Could you check a few things on this model? Use its own coordinates, in mm. Face numbers are marked on the shaded views. A direction names the side the tool comes from. Coordinates: 2 decimals unless noted, no trailing zeros. Loops run counter-clockwise (first coordinate to the right, second up) from the corner with the lowest first, then second, coordinate; pieces in that order, holes last. Notation, with made-up numbers: M 66.25,-13 L 89.25,-13 A23 ccw 89.25,1 Z; hole C -18,38.5 d4. An arc over 180 degrees is marked long. Return JSON: item names as keys, results as strings. Group by question number.
Autodesk Inventor part; units mm, degrees
ref_plane "Work Plane2" through (20.6375, 27.2274, 0) normal (-1, 0, 0) x (0, 0, -1)
ref_plane "YZ Plane" through (0, 0, 0) normal (1, 0, 0) x (0, 1, 0)
ref_plane "XZ Plane" through (0, 0, 0) normal (0, 1, 0) x (-1, 0, 0)
sketch "Sketch1" plane through (0, 0, 0) normal (0, 0, 1) x (1, 0, 0)
  circle A0 centre (0, 0) radius 20.2565
  dimension "d1" = 40.513
sketch "Sketch2" plane through (0, 0, 0) normal (1, 0, 0) x (0, 1, 0)
  line L0 (0, 0) -> (27.2274, 0)
  line L1 (27.2274, 0) -> (27.2274, -51.0956)
  line L2 (27.2274, -51.0956) -> (0, -51.0956)
  line L3 (0, -51.0956) -> (0, 0)
ref_plane "Work Plane2" through (20.6375, 27.2274, 0) normal (-1, 0, 0) x (0, 0, -1)
ref_plane "Work Plane1" through (0, 27.2274, 0) normal (-1, 0, 0) x (0, 0, -1)
extrude "Extrusion1" add sketch "Sketch1" against normal blind 52.0573
sketch "Sketch3" plane through (0, 0, 0) normal (0, 0, 1) x (1, 0, 0)
  circle A0 centre (0, 0) radius 16.7767
  dimension "d5" = 33.5534
sketch "Sketch4" plane through (20.6375, 27.2274, 0) normal (-1, 0, 0) x (0, 0, -1)
  line L0 (52.0573, 6.9709) -> (52.0573, 47.4839)
  circle A0 centre (52.0573, 27.2274) radius 20.2565
  point P0 (0, 27.2274)
sketch "Sketch5" plane through (20.6375, 27.2274, 0) normal (-1, 0, 0) x (0, 0, -1)
  circle A0 centre (52.1379, 27.2274) radius 16.7767
  point P0 (0, 27.2274)
  dimension "d10" = 33.5534
extrude "Extrusion2" add sketch "Sketch4" along normal blind 41.275
extrude "Extrusion3" cut sketch "Sketch5" along normal through all
extrude "Extrusion4" cut sketch "Sketch3" against normal blind 31.9024
properties part number "Slip Tee 1 Inch"
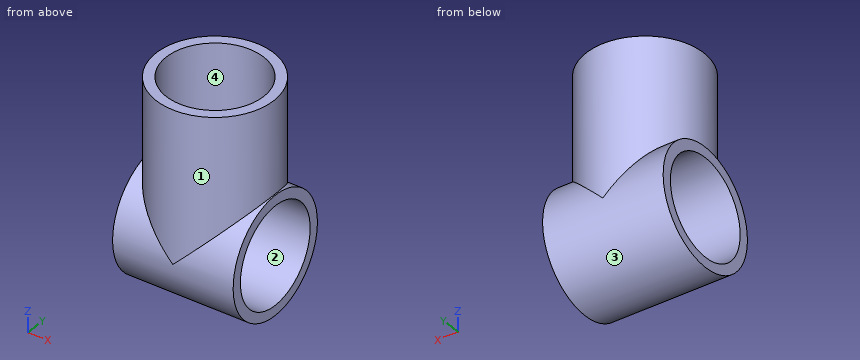
(1) Imagine slicing it at B-B, the plane x = 0. Write out the boundary of the cut face in (y, z), then the cut area to 3 significant figures.
(2) Will these pins go through, and if not, where does the flat tip stop? P1, Ø6, axis at x = 8, y = -0.5, coming from the +Z side; P2, Ø2, axis at x = 8.5, z = -41, coming from the -Y side; P3, Ø5, axis at x = 10, z = -38, coming from the +Y side.
(3) For the marked faces 3 and 4, which set-ups out of +Z, -Z, +X, -X, +Y, -Y let a thin tool reach every point of the face, with its end or its side?
(4) We'd pull the mould along Y, two halves only. Please class the marked faces 1 and 2: +Y half, -Y half, draft (parallel to the pull), parting line (faces both ways), or undercut.
(5) Imagine slicing it at A-A, the plane y = 0. Write out the boundary of the cut face in (x, z).
(6) If I drill on L1, parallel to Z at x = -11, y = 0; L2, parallel to Y at x = 16.5, z = -52.5, over which ranges is the centre line in solid material (lowest first)? Write a range as [from, to].
(7) Imagine slicing it at D-D, the plane z = -8. Write out the boundary of the cut face in (x, y).
(8) Imagine slicing it at C-C, the plane z = -40.5. Write out the boundary of the cut face in (x, y), then the cut area to 3 significant figures.
Checks:
{
 "1": {"outline": "M -20.26,-52.06 A20.26 ccw 20.26,-52.06 L 20.26,0 L 16.78,0 L 16.78,-31.9 L -16.78,-31.9 L -16.78,0 L -20.26,0 Z; hole C 0,-52.14 d33.55", "area": "799 mm²"},
 "2": {"P1": "z = -31.9", "P2": "y = -18.82", "P3": "y = 18.82"},
 "3": {"face 3": "none", "face 4": "+Z"},
 "4": {"face 1": "parting line", "face 2": "undercut"},
 "5": {"outline": "M -20.64,-72.31 L 20.64,-72.31 L 20.64,-68.91 L -20.64,-68.91 Z; M -20.64,-35.36 L 20.64,-35.36 L 20.64,-31.8 L 20.26,-31.8 L 20.26,0 L 16.78,0 L 16.78,-31.9 L -16.78,-31.9 L -16.78,0 L -20.26,0 L -20.26,-31.8 L -20.64,-31.8 Z"},
 "6": {"L1": "[-72.31, -68.91], [-35.36, -31.9]", "L2": "[-20.25, -16.77], [16.77, 20.25]"},
 "7": {"outline": "C 0,0 d40.51; hole C 0,0 d33.55"},
 "8": {"outline": "M -20.64,-16.64 L -11.56,-16.64 A20.26 ccw 11.56,-16.64 L 20.64,-16.64 L 20.64,-12.08 L -20.64,-12.08 Z; M -20.64,12.08 L 20.64,12.08 L 20.64,16.64 L 11.56,16.64 A20.26 ccw -11.56,16.64 L -20.64,16.64 Z", "area": "490 mm²"}
}
